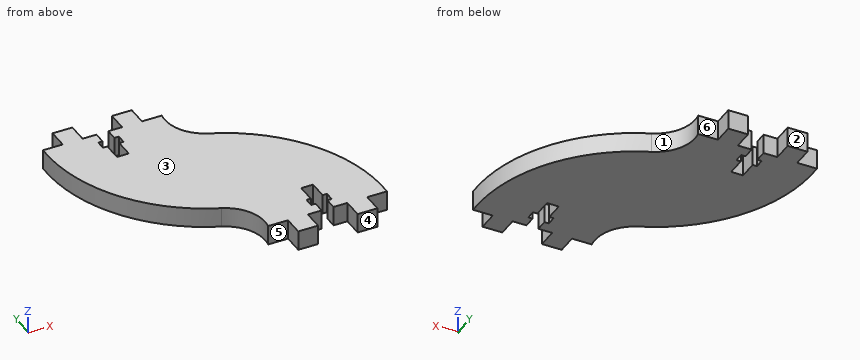
from build123d import *

# Parameters (mm, degrees)
BOSS_EXTRUDE1_DEPTH = 5


with BuildPart() as part:
    # Sketch1 → Boss-Extrude1 (new body)
    with BuildSketch(Plane.XY):
        with BuildLine():
            Line((-11, 50), (-6, 50))
            ThreePointArc((-6, 50), (-4.955689192, 43.335228836), (0.083613647, 38.850233113))
            ThreePointArc((0.083613647, 38.850233113), (18.735492032, 23.397402982), (25, 0))
            Line((25, 0), (20, 0))
            Line((20, 0), (20, -5))
            Line((20, -5), (15, -5))
            Line((15, -5), (15, 0))
            Line((15, 0), (11.5, 0))
            Line((11.5, 0), (11.5, 3))
            Line((11.5, 3), (12.6, 3))
            Line((12.6, 3), (12.6, 5.3))
            Line((12.6, 5.3), (11.5, 5.3))
            Line((11.5, 5.3), (11.5, 10))
            Line((11.5, 10), (8.5, 10))
            Line((8.5, 10), (8.5, 5.3))
            Line((8.5, 5.3), (7.4, 5.3))
            Line((7.4, 5.3), (7.4, 3))
            Line((7.4, 3), (8.5, 3))
            Line((8.5, 3), (8.5, 0))
            Line((8.5, 0), (5, 0))
            Line((5, 0), (5, -5))
            Line((5, -5), (0, -5))
            Line((0, -5), (0, 0))
            Line((0, 0), (-5, 0))
            ThreePointArc((-5, 0), (-6.044310808, 6.664771164), (-11.083613647, 11.149766887))
            ThreePointArc((-11.083613647, 11.149766887), (-29.735492032, 26.602597018), (-36, 50))
            Line((-36, 50), (-31, 50))
            Line((-31, 50), (-31, 55))
            Line((-31, 55), (-26, 55))
            Line((-26, 55), (-26, 50))
            Line((-26, 50), (-22.5, 50))
            Line((-22.5, 50), (-22.5, 47))
            Line((-22.5, 47), (-23.6, 47))
            Line((-23.6, 47), (-23.6, 44.7))
            Line((-23.6, 44.7), (-22.5, 44.7))
            Line((-22.5, 44.7), (-22.5, 40))
            Line((-22.5, 40), (-19.5, 40))
            Line((-19.5, 40), (-19.5, 44.7))
            Line((-19.5, 44.7), (-18.4, 44.7))
            Line((-18.4, 44.7), (-18.4, 47))
            Line((-18.4, 47), (-19.5, 47))
            Line((-19.5, 47), (-19.5, 50))
            Line((-19.5, 50), (-16, 50))
            Line((-16, 50), (-16, 55))
            Line((-16, 55), (-11, 55))
            Line((-11, 55), (-11, 50))
        make_face()
    extrude(amount=BOSS_EXTRUDE1_DEPTH)


solid = part.part
Verification items for the finished model (mm, model axes). Face numbers are marked on the shaded views. A direction names the side the tool comes from. Give positions to 0.01 mm unless a question says otherwise; leave off trailing zeros. Order: outer loops, then holes, each group sorted by start corner. A loop starts at its lowest first (then second) coordinate and runs counter-clockwise, first axis right, second up. Notation, with made-up numbers: (11, -14.75) -> (50, -14.75) arc R9 ccw to (50, -3.75) -> close; hole circle Ø3 at (79, 47.5). An arc over 180 degrees is marked (long way). Answer as CSV lines item,"result".
Q1. Release check for a two-part mould opening along Y. For the marked faces 1, 2 and 3 record: +Y half, -Y half, draft (parallel to the pull), parting line (faces both ways), or undercut.
Solutions:
face 1,"undercut"
face 2,"+Y half"
face 3,"draft"
Q2. Depth check by flat-ended pin: pin 1 (2.5 mm diameter, centred on y = 48, z = 3.5, fed in from +X); pin 2 (1.2 mm diameter, centred on x = -23, z = 3, fed in from +Y); pin 3 (2.5 mm diameter, centred on y = 49, z = 2, fed in from -X). Enter the tip coordinate at first touch or a pass-through.
Solutions:
pin 1,"stops at x = -6.08"
pin 2,"stops at y = 50"
pin 3,"stops at x = -36.04"
Q3. Sectioned sample at D-D on y = 23. Record the cut outline in (x, z), plus the area to 3 significant figures.
Solutions:
outline,"(-27.13, 0) -> (18.99, 0) -> (18.99, 5) -> (-27.13, 5) -> close"
area,"231 mm²"
Q4. Sectioned sample at C-C on y = 6.5. Record the cut outline in (x, z), plus the area to 3 significant figures.
Solutions:
outline,"(-5.96, 0) -> (8.5, 0) -> (8.5, 5) -> (-5.96, 5) -> close; (11.5, 0) -> (24.77, 0) -> (24.77, 5) -> (11.5, 5) -> close"
area,"139 mm²"
Q5. Sectioned sample at A-A on y = 51.5. Record the cut outline in (x, z).
Solutions:
outline,"(-31, 0) -> (-26, 0) -> (-26, 5) -> (-31, 5) -> close; (-16, 0) -> (-11, 0) -> (-11, 5) -> (-16, 5) -> close"
Q6. Sectioned sample at B-B on x = 17. Record the cut outline in (y, z).
Solutions:
outline,"(-5, 0) -> (25.89, 0) -> (25.89, 5) -> (-5, 5) -> close"
Q7. Access from +Z, -Z, +X, -X, +Y, -Y to the whole of each face (thin tool, end or side, straight path). Record for the marked faces 4, 5 and 6.
Solutions:
face 4,"+Z, -Z, +X, -X, -Y"
face 5,"+Z, -Z, -X, -Y"
face 6,"+Z, -Z, +X, +Y"
Q8. Scan lines: probe 1 along X at (y, z) = (5, 4.3); probe 2 along X at (y, z) = (8.5, 0.75); probe 3 along Y at (x, z) = (-9, 4.5). Record each from-to range of solid material in increasing order.
Solutions:
probe 1,"x = -5.32 to 7.4, 12.6 to 24.92"
probe 2,"x = -7.33 to 8.5, 11.5 to 24.49"
probe 3,"y = 10.01 to 50"
